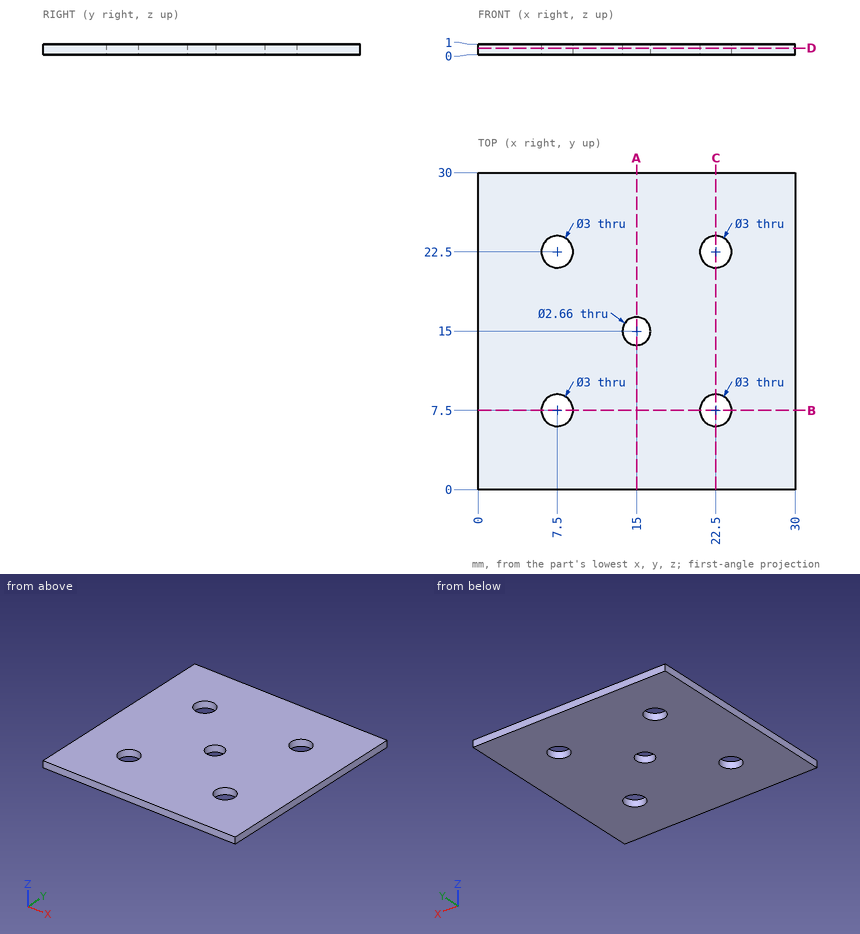
Geometry check sheet. Reference: drawing and pictorial views, mm from the part's lowest x, y, z. Give positions to 0.01 mm unless a question says otherwise; leave off trailing zeros. Order: outer loops, then holes, each group sorted by start corner. A loop starts at its lowest first (then second) coordinate and runs counter-clockwise, first axis right, second up. Notation, with made-up numbers: M 30,89 L 79,89 A20 ccw 79,93 Z; hole C -11.75,39.25 d1. An arc over 180 degrees is marked long. Use one line per item in the form item = value. Start each with the question number.
Q1. Section check A-A (x = 15). Enter the section's corners in (y, z).
Q2. Scan lines: line 1 along Y through (x, z) = (7.5, 0.2); line 2 along X through (y, z) = (22.75, 0.9); line 3 along Y through (x, z) = (15, 0.75). Record each from-to range of solid material in increasing order. Write a range as [from, to].
Q3. Section check D-D (z = 0.6). Enter the section's corners in (x, y), then the cut area to 3 significant figures.
Q4. Section check B-B (y = 7.5). Enter the section's corners in (x, z), then the cut area to 3 significant figures.
Evaluation:
q1.outline = M 0,0 L 13.67,0 L 13.67,1 L 0,1 Z; M 16.33,0 L 30,0 L 30,1 L 16.33,1 Z
q2.line_1 = [0, 6], [9, 21], [24, 30]
q2.line_2 = [0, 6.02], [8.98, 21.02], [23.98, 30]
q2.line_3 = [0, 13.67], [16.33, 30]
q3.outline = M 0,0 L 30,0 L 30,30 L 0,30 Z; hole C 7.5,7.5 d3; hole C 7.5,22.5 d3; hole C 15,15 d2.66; hole C 22.5,7.5 d3; hole C 22.5,22.5 d3
q3.area = 866 mm2
q4.outline = M 0,0 L 6,0 L 6,1 L 0,1 Z; M 9,0 L 21,0 L 21,1 L 9,1 Z; M 24,0 L 30,0 L 30,1 L 24,1 Z
q4.area = 24.0 mm2
